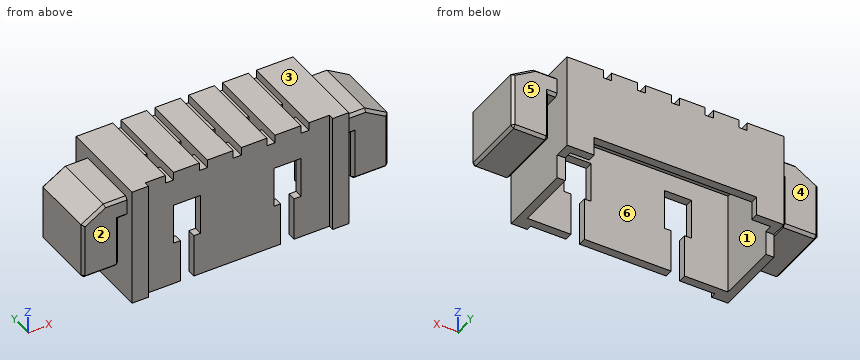
```python
from build123d import *

# Parameters (mm, degrees)
SKETCH1_W                = 8
SKETCH1_H                = 4.4
BOSS_EXTRUDE1_DEPTH      = 3.4
SKETCH4_W                = 6.8
SKETCH4_H                = 4.4
CUT_EXTRUDE1_DEPTH       = 0.2
SHELL1_START             = -3.7
SHELL1_OUTLINE_W         = 2.6
SHELL1_OUTLINE_H         = 4.1
SHELL1_DEPTH             = 7.4
CUT_EXTRUDE3_REACH       = 8.85
SKETCH8_W                = 7.4
SKETCH8_H                = 2.6
BOSS_EXTRUDE2_DEPTH      = 0.3
SKETCH3_3_W              = 0.3
SKETCH3_3_H              = 1.4
CUT_EXTRUDE4_DEPTH       = 7.849817516
SKETCH9_W                = 0.3
SKETCH9_H                = 0.8
CUT_EXTRUDE5_DEPTH       = 7.849817516
SKETCH10_W               = 8
SKETCH10_H               = 0.9
CUT_EXTRUDE6_DEPTH       = 0.6
SKETCH11_W               = 6
SKETCH11_H               = 0.7
CUT_EXTRUDE7_DEPTH       = 1
BOSS_EXTRUDE3_START      = -0.3
BOSS_EXTRUDE3_DEPTH      = 2.5
CHAMFER1_SIZE            = 0.1
CHAMFER1_OF_MIRROR2_SIZE = 0.1


# Read off the part's stored shape, not the designer's step: Shell1
with BuildPart() as part:
    # Sketch1 → Boss-Extrude1 (new body)
    with BuildSketch(Plane(origin=(0, 0, 0), x_dir=(1, 0, 0), z_dir=(0, 1, 0))):
        with Locations((0, -2.2)):
            Rectangle(SKETCH1_W, SKETCH1_H)
    extrude(amount=BOSS_EXTRUDE1_DEPTH)

    # Sketch4 → Cut-Extrude1 (cut)
    with BuildSketch(Plane.XZ):
        with Locations((0, 2.2)):
            Rectangle(SKETCH4_W, SKETCH4_H)
    extrude(amount=-CUT_EXTRUDE1_DEPTH, mode=Mode.SUBTRACT)

    # Shell1 outline → Shell1 (cut)
    with BuildSketch(Plane.YZ.offset(SHELL1_START)):
        with Locations((1.8, 2.05)):
            Rectangle(SHELL1_OUTLINE_W, SHELL1_OUTLINE_H)
    extrude(amount=SHELL1_DEPTH, mode=Mode.SUBTRACT)

    # Sketch3 → Cut-Extrude3 (cut, up to next)
    with BuildSketch(Plane(origin=(0, 0, 0), x_dir=(1, 0, 0), z_dir=(0, 1, 0)), mode=Mode.PRIVATE) as cut_extrude3_sk1:
        Polygon((-1.6, -1.6), (-1.6, 0), (-2.1, 0), (-2.1, -1.6), (-2.35, -1.6), (-2.35, -3.1), (-1.35, -3.1), (-1.35, -1.6), align=None)
    cut_extrude3_tool1 = extrude(cut_extrude3_sk1.sketch, amount=CUT_EXTRUDE3_REACH, mode=Mode.PRIVATE) & part.part
    cut_extrude3 = cut_extrude3_tool1.solids().sort_by_distance((-1.85, 0, 1.81087))[0]
    add(cut_extrude3, mode=Mode.SUBTRACT)

    # Mirror1: Cut-Extrude3 across plane
    add(cut_extrude3.mirror(Plane(origin=(0, 0, 0), x_dir=(0, 0, 1), z_dir=(1, 0, 0))), mode=Mode.SUBTRACT)

    # Sketch8 → Boss-Extrude2 (add)
    with BuildSketch(Plane(origin=(0, 0, 4.1), x_dir=(-1, 0, 0), z_dir=(0, 0, -1))):
        with Locations((0, 1.8)):
            Rectangle(SKETCH8_W, SKETCH8_H)
    extrude(amount=BOSS_EXTRUDE2_DEPTH)

    # Sketch3<3> → Cut-Extrude4 (cut, through all)
    with BuildSketch(Plane(origin=(0, 0, 0), x_dir=(1, 0, 0), z_dir=(0, 1, 0))):
        with Locations((-2.5, -4.8)):
            Rectangle(SKETCH3_3_W, SKETCH3_3_H)
        with Locations((-1.25, -4.8)):
            Rectangle(SKETCH3_3_W, SKETCH3_3_H)
        with Locations((0, -4.8)):
            Rectangle(SKETCH3_3_W, SKETCH3_3_H)
        with Locations((1.25, -4.8)):
            Rectangle(SKETCH3_3_W, SKETCH3_3_H)
        with Locations((2.5, -4.8)):
            Rectangle(SKETCH3_3_W, SKETCH3_3_H)
    extrude(amount=CUT_EXTRUDE4_DEPTH, mode=Mode.SUBTRACT)

    # Sketch9 → Cut-Extrude5 (cut, through all)
    with BuildSketch(Plane.XY):
        with Locations((-2.5, 1.4)):
            Rectangle(SKETCH9_W, SKETCH9_H)
        with Locations((-1.25, 1.4)):
            Rectangle(SKETCH9_W, SKETCH9_H)
        with Locations((0, 1.4)):
            Rectangle(SKETCH9_W, SKETCH9_H)
        with Locations((1.25, 1.4)):
            Rectangle(SKETCH9_W, SKETCH9_H)
        with Locations((2.5, 1.4)):
            Rectangle(SKETCH9_W, SKETCH9_H)
    extrude(amount=CUT_EXTRUDE5_DEPTH, mode=Mode.SUBTRACT)

    # Sketch10 → Cut-Extrude6 (cut)
    with BuildSketch(Plane(origin=(0, 3.4, 0), x_dir=(1, 0, 0), z_dir=(0, 1, 0))):
        with Locations((0, -0.45)):
            Rectangle(SKETCH10_W, SKETCH10_H)
    extrude(amount=-CUT_EXTRUDE6_DEPTH, mode=Mode.SUBTRACT)

    # Sketch11 → Cut-Extrude7 (cut)
    with BuildSketch(Plane(origin=(0, 3.4, 0), x_dir=(1, 0, 0), z_dir=(0, 1, 0))):
        with Locations((0, -1.25)):
            Rectangle(SKETCH11_W, SKETCH11_H)
    extrude(amount=-CUT_EXTRUDE7_DEPTH, mode=Mode.SUBTRACT)

    # Sketch12 → Boss-Extrude3 (add)
    with BuildSketch(Plane.XZ.offset(BOSS_EXTRUDE3_START)):
        Polygon((4, 4), (4.825, 4), (5.65, 3.5), (5.65, 1.4), (4.3, 1.4), (4.3, 3.25), (4, 3.25), align=None)
    boss_extrude3 = extrude(amount=-BOSS_EXTRUDE3_DEPTH)

    # Chamfer1
    chamfer1_edges = [part.edges().sort_by_distance(p)[0] for p in [
        (4.4125, 2.8, 4),
        (5.2375, 2.8, 3.75),
        (5.65, 2.8, 2.45),
        (4.975, 2.8, 1.4),
        (5.65, 1.55, 1.4),
        (4.3, 2.8, 2.325),
        (4.3, 1.55, 1.4),
        (4.15, 2.8, 3.25),
        (4.15, 0.3, 3.25),
        (4.3, 0.3, 2.325),
        (4.975, 0.3, 1.4),
        (5.65, 0.3, 2.45),
        (5.2375, 0.3, 3.75),
        (4.4125, 0.3, 4),
    ]]
    chamfer(chamfer1_edges, length=CHAMFER1_SIZE)

    # Mirror2: Boss-Extrude3 across plane
    add(boss_extrude3.mirror(Plane(origin=(0, 0, 0), x_dir=(0, 0, 1), z_dir=(1, 0, 0))))

    # Chamfer1 of Mirror2
    chamfer1_of_mirror2_edges = [part.edges().sort_by_distance(p)[0] for p in [
        (-4.4125, 2.8, 4),
        (-5.2375, 2.8, 3.75),
        (-5.65, 2.8, 2.45),
        (-4.975, 2.8, 1.4),
        (-5.65, 1.55, 1.4),
        (-4.3, 2.8, 2.325),
        (-4.3, 1.55, 1.4),
        (-4.15, 2.8, 3.25),
        (-4.15, 0.3, 3.25),
        (-4.3, 0.3, 2.325),
        (-4.975, 0.3, 1.4),
        (-5.65, 0.3, 2.45),
        (-5.2375, 0.3, 3.75),
        (-4.4125, 0.3, 4),
    ]]
    chamfer(chamfer1_of_mirror2_edges, length=CHAMFER1_OF_MIRROR2_SIZE)


solid = part.part
```
Design review of the part built by this model. Coordinates are the model's own, in mm. Face numbers are marked on the shaded views. A direction names the side the tool comes from. Give positions to 0.01 mm unless a question says otherwise; leave off trailing zeros. Loops run counter-clockwise (first coordinate to the right, second up) from the corner with the lowest first, then second, coordinate; pieces in that order, holes last. Notation, with made-up numbers: M -33.75,79.25 L -25.75,79.25 A24 ccw -25.75,114.25 Z; hole C -30.75,58.5 d3. An arc over 180 degrees is marked long. Return JSON: item names as keys, results as strings. Group by question number.
Item 1: We need section B-B (z = 0.55). Give the boundary of the cut face in (x, y).
Item 2: We need section C-C (y = 1.4). Give the number of separate pieces and of enclosed holes in the cut face, and give its area (3 significant figures).
Item 3: We need section A-A (x = 0). Give the boundary of the cut face in (y, z).
Item 4: Mouldability with a two-part tool opening along Y and no side actions: class the marked faces 1, 2 and 3 as released by +Y, released by -Y, zero draft, split by the parting line, or undercut.
Item 5: For probe 1 along X at (y, z) = (2.05, 3.2); probe 2 along Y at (x, z) = (3.5, 1.25); probe 3 along X at (y, z) = (0.9, 1.1), list the stretches that pass through material, from the lowest coordinate up.
Item 6: Insertion check: pin 1 Ø0.5 at (y, z) = (1.5, 4) entering from +X; pin 2 Ø0.8 at (x, z) = (-4.5, 3) entering from +Y. Each pin has a flat end and moves straight along its axis. Give the tip position at first contact, or say it passes through.
Item 7: Tool access review of the marked faces 4, 5 and 6: name each direction out of +Z, -Z, +X, -X, +Y, -Y from which nothing blocks a thin tool from reaching the whole face with its end or side.
Output:
{
 "1": {"outline": "M -4,0 L -3.4,0 L -3.4,0.2 L -2.1,0.2 L -2.1,0.5 L -3.7,0.5 L -3.7,2.8 L -4,2.8 Z; M -1.6,0.2 L 1.6,0.2 L 1.6,0.5 L -1.6,0.5 Z; M 2.1,0.2 L 3.4,0.2 L 3.4,0 L 4,0 L 4,2.8 L 3.7,2.8 L 3.7,0.5 L 2.1,0.5 Z"},
 "2": {"separate pieces": "6", "enclosed holes": "0", "area": "13.2 mm^2"},
 "3": {"outline": "M 0.2,0 L 0.5,0 L 0.5,3.8 L 1,3.8 L 1,4.1 L 0.2,4.1 Z; M 1.8,3.8 L 3.1,3.8 L 3.1,1.6 L 3.4,1.6 L 3.4,4.1 L 1.8,4.1 Z"},
 "4": {"face 1": "undercut", "face 2": "released by -Y", "face 3": "zero draft"},
 "5": {"probe 1": "x = -5.65 to -4.3, -4 to -3.7, 3.7 to 4, 4.3 to 5.65", "probe 2": "y = 0 to 0.5, 3.1 to 3.4", "probe 3": "x = -4 to -3.7, 3.7 to 4"},
 "6": {"pin 1": "stops at x = 5.24", "pin 2": "stops at y = 2.8"},
 "7": {"face 4": "+Z, -Z, -X, +Y", "face 5": "+Z, -Z, +X, +Y", "face 6": "-Z"}
}
